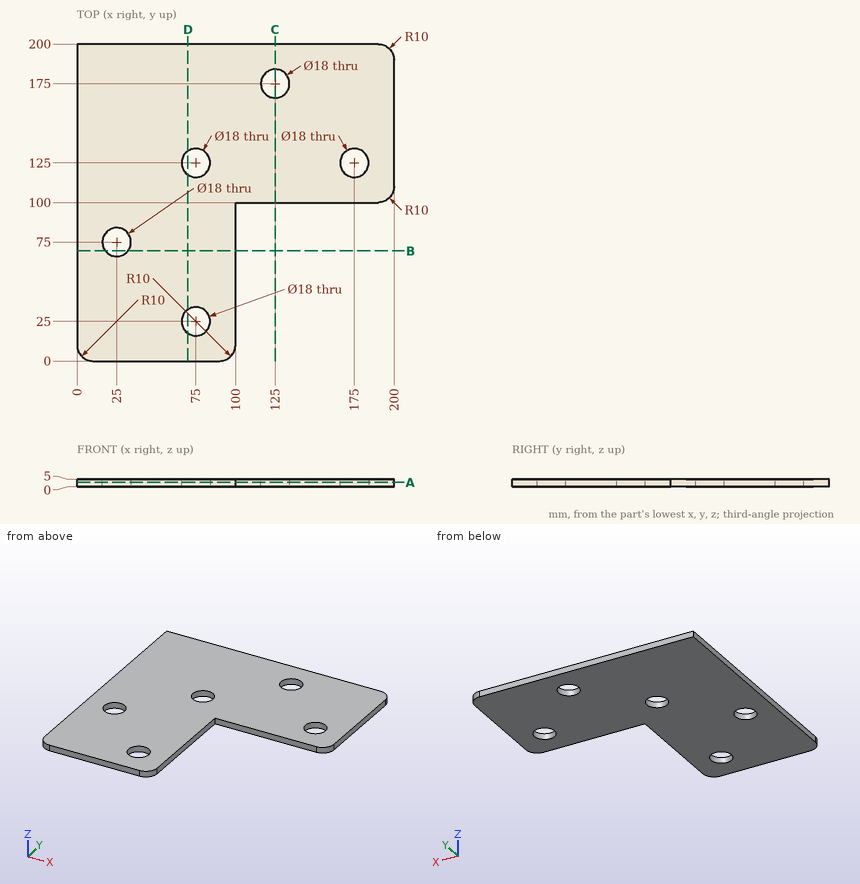
For this review, use the dimensioned drawing (mm, ordinates from the lowest corner) and the shaded views. Round coordinates to 2 decimals unless told otherwise and drop trailing zeros. Write each loop counter-clockwise with the first axis right and the second up, starting at its lowest first coordinate (ties: lowest second). Pieces come first, ordered by that corner, then holes. Notation, with made-up numbers: (-26, -26.5) -> (10, -26.5) arc R22 ccw to (10, 4.5) -> close; hole circle Ø8 at (2.5, 14). An arc over 180 degrees is marked (long way). Use one line per item in the form item = value.
Q1. Consider section D-D (x = 70). State the section outline as (y, z) points.
Resolved:
outline = (0, 0) -> (17.52, 0) -> (17.52, 5) -> (0, 5) -> close; (32.48, 0) -> (117.52, 0) -> (117.52, 5) -> (32.48, 5) -> close; (132.48, 0) -> (200, 0) -> (200, 5) -> (132.48, 5) -> close
Q2. Clearance check with flat-ended pins moving along their axes: pin 1 Ø20.5 at (x, y) = (175, 125) entering from -Z; pin 2 Ø1.5 at (x, z) = (161, 1.5) entering from -Y; pin 3 Ø14.5 at (x, y) = (75, 125) entering from -Z; pin 4 Ø1.5 at (y, z) = (63, 1.5) entering from +X. State where each tip first meets the part, or that it passes through.
Resolved:
pin_1 = 0
pin_2 = 100
pin_3 = through
pin_4 = 100
Q3. To check wall thickness, follow probe 1 along X at (y, z) = (124, 0.5); probe 2 along Y at (x, z) = (76, 4.5); probe 3 along Y at (x, z) = (24, 4.55). State the ranges of each line that lie inside material, in increasing order. Write a range as from..to.
Resolved:
probe_1 = 0..66.06, 83.94..166.06, 183.94..200
probe_2 = 0..16.06, 33.94..116.06, 133.94..200
probe_3 = 0..66.06, 83.94..200
Q4. Consider section A-A (z = 2.8). State the section outline as (x, y) points, then the cut area to 3 significant figures.
Resolved:
outline = (0, 10) arc R10 ccw to (10, 0) -> (90, 0) arc R10 ccw to (100, 10) -> (100, 100) -> (190, 100) arc R10 ccw to (200, 110) -> (200, 190) arc R10 ccw to (190, 200) -> (0, 200) -> close; hole circle Ø18 at (25, 75); hole circle Ø18 at (75, 25); hole circle Ø18 at (75, 125); hole circle Ø18 at (125, 175); hole circle Ø18 at (175, 125)
area = 28,600 mm²
Q5. Consider section B-B (y = 69.5). State the section outline as (x, z) points.
Resolved:
outline = (0, 0) -> (17.88, 0) -> (17.88, 5) -> (0, 5) -> close; (32.12, 0) -> (100, 0) -> (100, 5) -> (32.12, 5) -> close
Q6. Consider section C-C (x = 125). State the section outline as (y, z) points.
Resolved:
outline = (100, 0) -> (166, 0) -> (166, 5) -> (100, 5) -> close; (184, 0) -> (200, 0) -> (200, 5) -> (184, 5) -> close
